Here's how the part is built. I have some questions about the finished solid (model axes, mm). Coordinates: 2 decimals unless noted, no trailing zeros. Write each loop counter-clockwise with the first axis right and the second up, starting at its lowest first coordinate (ties: lowest second). Pieces come first, ordered by that corner, then holes. Notation, with made-up numbers: (-27, 57) -> (-11, 57) arc R25 cw to (-11, 74) -> close; hole circle Ø3 at (-35, 47). An arc over 180 degrees is marked (long way). Answer in a Markdown table with one row per item. Add a question column.
from build123d import *


with BuildPart() as part:
    # Sketch2 → Revolve1 (revolve)
    with BuildSketch(Plane(origin=(0, 0, 0), x_dir=(0, 0, -1), z_dir=(1, 0, 0))):
        with BuildLine():
            Line((-4.15, -1.9), (-4.15, 0))
            Line((-4.15, 0), (-2.752124344, 0))
            ThreePointArc((-2.752124344, 0), (-2.575, 0.822875656), (-2.075, 1.5))
            Line((-2.075, 1.5), (-1.75, 1.5))
            Line((-1.75, 1.5), (-1.75, 1.2))
            Line((-1.75, 1.2), (-2.211946903, 0))
            Line((-2.211946903, 0), (-2.211946903, -1.26))
            Line((-2.211946903, -1.26), (-1.75, -2.13))
            Line((-1.75, -2.13), (-2.25, -2.63))
            Line((-2.25, -2.63), (-2.85, -1.5))
            Line((-2.85, -1.5), (-3.3, -1.5))
            Line((-3.3, -1.5), (-3.85, -3))
            Line((-3.85, -3), (-4.55, -3))
            Line((-4.55, -3), (-4.15, -1.9))
        make_face()
    revolve(axis=Axis((0, 0, 0), (0, 1, 0)))


solid = part.part
Q1. Imagine slicing it at A-A on y = -2.45. Please give me the cut outline in (x, z), plus the area to 3 significant figures.
Q2. I'm going to push flat-ended pins straight in: P1, Ø5, axis at x = 0, z = 0, coming from the -Y side; P2, Ø1.5, axis at x = 2.5, y = -2.5, coming from the +Z side; P3, Ø1.5, axis at x = -2.5, y = -2, coming from the +Z side. Where does each tip first touch, or does it pass through?
Q3. If we mould it in two halves opening along Y, with no side actions, what happens to faces 1 (the cylindrical face through (-1.55, 1.35, 0.81)), 2 (the flat face through (1, -3, 4)), 3 (the flat face through (-3, 0, 1)), 4 (the cylindrical face through (0.7, -0.6, 2.1))? For each: pulls with the +Y half, pulls with the -Y half, needs draft (parallel to the pull), parting line crosses it, or undercut.
Q4. I need wall thicknesses on line 1 (Z direction, x = 1.5, y = -2.1); line 2 (X direction, y = -1.9, z = -2); line 3 (X direction, y = 1.45, z = 0). Which ranges of each line are inside material? Lowest first, please. Write a range as [from, to].
Q5. Imagine slicing it at B-B on y = -0.8. Please give me the cut outline in (x, z), plus the area to 3 significant figures.
Result sheet:
| question | item | result |
|---|---|---|
| 1 | outline | circle Ø8.7 at (0, 0); circle Ø4.69 at (0, 0); hole circle Ø7.3 at (0, 0); hole circle Ø4.14 at (0, 0) |
| 1 | area | 21.5 mm^2 |
| 2 | P1 | stops at y = -2.63 |
| 2 | P2 | stops at z = 4.12 |
| 2 | P3 | stops at z = 3.91 |
| 3 | face 1 | needs draft |
| 3 | face 2 | pulls with the -Y half |
| 3 | face 3 | pulls with the +Y half |
| 3 | face 4 | undercut |
| 4 | line 1 | z = [-3.95, -3.18], [-2.04, -0.93], [0.93, 2.04], [3.18, 3.95] |
| 4 | line 2 | x = [-3.64, -2.81], [-1.72, 1.72], [2.81, 3.64] |
| 4 | line 3 | x = [-2.13, -1.75], [1.75, 2.13] |
| 5 | outline | circle Ø8.3 at (0, 0); hole circle Ø4.42 at (0, 0) |
| 5 | area | 38.7 mm^2 |
